from build123d import *

# Parameters (mm, degrees)
SKETCH10_R                                     = 2.5
BOSS_EXTRUDE2_DEPTH                            = 6.35
CBORE_FOR_4_SOCKET_HEAD_CAP_SCREW1_D           = 3.2639
CBORE_FOR_4_SOCKET_HEAD_CAP_SCREW1_CBORE_D     = 5.55752
CBORE_FOR_4_SOCKET_HEAD_CAP_SCREW1_CBORE_DEPTH = 2.8448
BOSS_EXTRUDE3_START                            = 6.35
BOSS_EXTRUDE3_DEPTH                            = 15
BOSS_EXTRUDE6_START                            = 6.35
BOSS_EXTRUDE6_DEPTH                            = 3.175


with BuildPart() as part:
    # Sketch10 → Boss-Extrude2 (new body)
    # profile 1 of 10: a face of its own
    with BuildSketch(Plane.XY):
        Polygon((180, 10), (0, 10), (0, 0), (55.075212776, 0), (62.146280588, 0), (64.974707713, 0), (72.045775525, 0), (170, 0), (170, -65), (137.045775525, -65), (129.974707713, -65), (128, -65), (128, -141.2), (52, -141.2), (52, -65), (0, -65), (0, -75), (42, -75), (42, -151.2), (138, -151.2), (138, -75), (180, -75), align=None)
    # profile 2 of 10: a face of its own
    with BuildSketch(Plane.XY):
        Polygon((0, 13.175), (0, 10), (180, 10), (180, -75), (138, -75), (138, -151.2), (42, -151.2), (42, -75), (0, -75), (0, -78.175), (38.825, -78.175), (38.825, -154.375), (141.175, -154.375), (141.175, -78.175), (183.175, -78.175), (183.175, 13.175), align=None)
    # profile 3 of 10: a face of its own
    with BuildSketch(Plane.XY):
        Polygon((55.075212776, 0), (0, 0), (0, -65), (52, -65), (52, -141.2), (128, -141.2), (128, -65), (127.146280588, -65), (120.075212776, -65), (57.075212776, -2), align=None)
        with Locations((66.974707713, -119.977801383)):
            Circle(SKETCH10_R, mode=Mode.SUBTRACT)
    # profile 4 of 10: a face of its own
    with BuildSketch(Plane.XY):
        Polygon((62.146280588, 0), (55.075212776, 0), (57.075212776, -2), (64.146280588, -2), align=None)
    # profile 5 of 10: a face of its own
    with BuildSketch(Plane.XY):
        Polygon((64.974707713, 0), (62.146280588, 0), (64.146280588, -2), (127.146280588, -65), (128, -65), (129.974707713, -65), (127.974707713, -63), (66.974707713, -2), align=None)
    # profile 6 of 10: a face of its own
    with BuildSketch(Plane.XY):
        Polygon((64.146280588, -2), (57.075212776, -2), (120.075212776, -65), (127.146280588, -65), align=None)
    # profile 7 of 10: a face of its own
    with BuildSketch(Plane.XY):
        Polygon((72.045775525, 0), (64.974707713, 0), (66.974707713, -2), (74.045775525, -2), align=None)
    # profile 8 of 10: a face of its own
    with BuildSketch(Plane.XY):
        Polygon((170, 0), (72.045775525, 0), (74.045775525, -2), (135.045775525, -63), (137.045775525, -65), (170, -65), align=None)
    # profile 9 of 10: a face of its own
    with BuildSketch(Plane.XY):
        Polygon((74.045775525, -2), (66.974707713, -2), (127.974707713, -63), (135.045775525, -63), align=None)
    # profile 10 of 10: a face of its own
    with BuildSketch(Plane.XY):
        Polygon((135.045775525, -63), (127.974707713, -63), (129.974707713, -65), (137.045775525, -65), align=None)
    extrude(amount=BOSS_EXTRUDE2_DEPTH)

    # CBORE for #4 Socket Head Cap Screw1 (through all)
    with Locations(Plane(origin=(4.3688, 5, 6.35), x_dir=(1, 0, 0), z_dir=(0, 0, 1))):
        with Locations((0, 0), (34.12624, 0), (68.25248, 0), (102.37872, 0), (136.50496, 0), (170.6312, 0), (170.6312, -75), (128.6312, -75), (128.6312, -113.1), (128.6312, -151.2), (85.6312, -151.2), (42.6312, -151.2), (42.6312, -113.1), (42.6312, -75), (0, -75)):
            CounterBoreHole(CBORE_FOR_4_SOCKET_HEAD_CAP_SCREW1_D / 2, CBORE_FOR_4_SOCKET_HEAD_CAP_SCREW1_CBORE_D / 2, CBORE_FOR_4_SOCKET_HEAD_CAP_SCREW1_CBORE_DEPTH)



with BuildPart() as body_2:
    # Sketch13 → Boss-Extrude3 (new body)
    with BuildSketch(Plane.XY.offset(BOSS_EXTRUDE3_START)):
        Polygon((187.35, 17.35), (0, 17.35), (0, 13.675), (183.675, 13.675), (183.675, -78.675), (141.675, -78.675), (141.675, -154.875), (38.325, -154.875), (38.325, -78.675), (0, -78.675), (0, -81.85), (35.15, -81.85), (35.15, -158.05), (144.85, -158.05), (144.85, -81.85), (187.35, -81.85), align=None)
    extrude(amount=-BOSS_EXTRUDE3_DEPTH)


with BuildPart() as part_1:
    add(part.part)

    add(body_2.part)  # Boss-Extrude6 merges body 2
    # Sketch13<7> → Boss-Extrude6 (add)
    with BuildSketch(Plane.XY.offset(BOSS_EXTRUDE6_START)):
        Polygon((138, -75), (180, -75), (180, 10), (0, 10), (0, 13.175), (183.175, 13.175), (183.175, -78.175), (141.175, -78.175), (141.175, -154.375), (38.825, -154.375), (38.825, -78.175), (0, -78.175), (0, -75), (42, -75), (42, -151.2), (138, -151.2), align=None)
        Polygon((183.175, 13.175), (0, 13.175), (0, 13.675), (183.675, 13.675), (183.675, -78.675), (141.675, -78.675), (141.675, -154.875), (38.325, -154.875), (38.325, -78.675), (0, -78.675), (0, -78.175), (38.825, -78.175), (38.825, -154.375), (141.175, -154.375), (141.175, -78.175), (183.175, -78.175), align=None)
    extrude(amount=-BOSS_EXTRUDE6_DEPTH)


solid = part_1.part
Could you check a few things on this model? Use its own coordinates, in mm. A direction names the side the tool comes from. Give positions to 0.01 mm unless a question says otherwise; leave off trailing zeros. Order: outer loops, then holes, each group sorted by start corner. A loop starts at its lowest first (then second) coordinate and runs counter-clockwise, first axis right, second up.
Item 1: If we section it at B-B, the plane y = -135: Write out the boundary of the cut face in (x, z) (3 decimals), plus the area to 3 significant figures.
Item 2: I need wall thicknesses on line 1 (X direction, y = -146.2, z = 5.7); line 2 (X direction, y = -108.1, z = 2.15) (3 decimals); line 3 (X direction, y = -91.5, z = 1.25) (3 decimals). Which ranges of each line are inside material? Lowest first, please.
Item 3: If we section it at A-A, the plane z = -3.5: Write out the boundary of the cut face in (x, y) (3 decimals), plus the area to 3 significant figures.
Item 4: If we mould it in two halves opening along Y, with no side actions, what happens to faces 4 (the face through (0, -32, 4)), 5 (the face through (107, 3, 3.505))? For each: pulls with the +Y half, pulls with the -Y half, needs draft (parallel to the pull), parting line crosses it, or undercut.
Item 5: I'm going to push flat-ended pins straight in: pin 1 (5 mm diameter, centred on x = 72.62, y = 5, fed in from +Z); pin 2 (4 mm diameter, centred on y = -94.5, z = -4, fed in from +X); pin 3 (1.5 mm diameter, centred on x = 156, y = -32, fed in from -Z). Where does each tip first touch, or does it pass through?
Item 6: For faces 1 (the face through (38.325, -117, -3)), 2 (the face through (90, -148, 3.505)), 3 (the face through (35.15, -119, -1)), which set-ups out of +Z, -Z, +X, -X, +Y, -Y let a thin tool reach every point of the face, with its end or its side?
Item 7: If we section it at C-C, the plane x = 25.5: Write out the boundary of the cut face in (y, z) (3 decimals).
Item 8: If we section it at D-D, the plane y = -26: Write out the boundary of the cut face in (x, z) (3 decimals), plus the area to 3 significant figures.
Values:
1. outline: (35.15, -8.65) - (38.325, -8.65) - (38.325, 3.175) - (38.825, 3.175) - (38.825, 0) - (141.175, 0) - (141.175, 3.175) - (141.675, 3.175) - (141.675, -8.65) - (144.85, -8.65) - (144.85, 6.35) - (35.15, 6.35) - close
1. area: 748 mm2
2. line 1: x = 35.15 to 44.22, 49.78 to 87.22, 92.78 to 130.22, 135.78 to 144.85
2. line 2: x = 35.15 to 38.325, 38.825 to 45.368, 48.632 to 131.368, 134.632 to 141.175, 141.675 to 144.85
2. line 3: x = 35.15 to 38.325, 38.825 to 141.175, 141.675 to 144.85
3. outline: (0, -81.85) - (35.15, -81.85) - (35.15, -158.05) - (144.85, -158.05) - (144.85, -81.85) - (187.35, -81.85) - (187.35, 17.35) - (0, 17.35) - (0, 13.675) - (183.675, 13.675) - (183.675, -78.675) - (141.675, -78.675) - (141.675, -154.875) - (38.325, -154.875) - (38.325, -78.675) - (0, -78.675) - close
3. area: 2,110 mm2
4. face 4: needs draft
4. face 5: undercut
5. pin 1: stops at z = 3.51
5. pin 2: stops at x = 144.85
5. pin 3: stops at z = 0
6. face 1: -Z
6. face 2: +Z
6. face 3: +Z, -Z, -X, -Y
7. outline: (-81.85, -8.65) - (-78.675, -8.65) - (-78.675, 3.175) - (-78.175, 3.175) - (-78.175, 0) - (13.175, 0) - (13.175, 3.175) - (13.675, 3.175) - (13.675, -8.65) - (17.35, -8.65) - (17.35, 6.35) - (-81.85, 6.35) - close
8. outline: (0, 0) - (183.175, 0) - (183.175, 3.175) - (183.675, 3.175) - (183.675, -8.65) - (187.35, -8.65) - (187.35, 6.35) - (0, 6.35) - close
8. area: 1,220 mm2
